```python
from build123d import *

# Parameters (mm, degrees)
SKETCH_W     = 58
SKETCH_H     = 40
PAD_DEPTH    = 2
SKETCH001_R  = 1.5
PAD001_DEPTH = 2
FILLET_R     = 3
SKETCH002_R  = 1.5
PAD002_DEPTH = 2
FILLET001_R  = 3


with BuildPart() as part:
    # Sketch → Pad (new body)
    with BuildSketch(Plane.XY):
        Rectangle(SKETCH_W, SKETCH_H)
    extrude(amount=PAD_DEPTH)

    # Sketch001 (on Face4 of Pad) → Pad001 (join)
    with BuildSketch(Plane(origin=(-29, 0, 0), x_dir=(0, -1, 0), z_dir=(-1, 0, 0))):
        with BuildLine():
            Line((-32.5, 2), (32.5, 2))
            ThreePointArc((32.5, -8), (37.5, -3), (32.5, 2))
            Line((-32.5, -8), (32.5, -8))
            ThreePointArc((-32.5, 2), (-37.5, -3), (-32.5, -8))
        make_face()
        with Locations((-32.5, -3)):
            Circle(SKETCH001_R, mode=Mode.SUBTRACT)
        with Locations((32.5, -3)):
            Circle(SKETCH001_R, mode=Mode.SUBTRACT)
    extrude(amount=PAD001_DEPTH)

    # Fillet
    fillet_edges = [part.edges().sort_by_distance(p)[0] for p in [
        (-29, 0, 0),
    ]]
    fillet(fillet_edges, radius=FILLET_R)

    # Sketch002 (on Face12 of Fillet) → Pad002 (join)
    with BuildSketch(Plane.YZ.offset(29)):
        with BuildLine():
            Line((-32.5, 2), (32.5, 2))
            ThreePointArc((32.5, -8), (37.5, -3), (32.5, 2))
            Line((-32.5, -8), (32.5, -8))
            ThreePointArc((-32.5, 2), (-37.5, -3), (-32.5, -8))
        make_face()
        with Locations((-32.5, -3)):
            Circle(SKETCH002_R, mode=Mode.SUBTRACT)
        with Locations((32.5, -3)):
            Circle(SKETCH002_R, mode=Mode.SUBTRACT)
    extrude(amount=PAD002_DEPTH)

    # Fillet001
    fillet001_edges = [part.edges().sort_by_distance(p)[0] for p in [
        (29, 0, 0),
    ]]
    fillet(fillet001_edges, radius=FILLET001_R)


solid = part.part
```
Geometry: final body of the model. Coordinates: model frame, mm. A direction names the side the tool comes from. Round coordinates to 2 decimals unless told otherwise and drop trailing zeros. Loops run counter-clockwise (first coordinate to the right, second up) from the corner with the lowest first, then second, coordinate; pieces in that order, holes last. Notation, with made-up numbers: (54.5, 27.5) -> (105.5, 27.5) arc R14 ccw to (105.5, 41.5) -> close; hole circle Ø2 at (39.5, 64.5). An arc over 180 degrees is marked (long way). Write each question's results on one line, items separated by ' | '.
Item 1: Set-up query: faces 1 (the face through (-30, -37.5, -3.1)), 2 (the face through (29, 1, -4)), 3 (the face through (0, 20, 1)), 4 (the face through (-28.14, 0.28, -0.9)). Return all of +Z, -Z, +X, -X, +Y, -Y with unobstructed straight access to the full face (end or side cutting, diameter ignored); none if empty.
Answers below:
face 1: +X, -X, -Y | face 2: -Z | face 3: +Z, -Z, +Y | face 4: -Z, +Y, -Y
Item 2: Cut plane A-A on y = 21.5. Return the cut outline in (x, z).
Answers below:
outline: (-31, -8) -> (-29, -8) -> (-29, 2) -> (-31, 2) -> close; (29, -8) -> (31, -8) -> (31, 2) -> (29, 2) -> close
Item 3: Line query: probe 1 along X at (y, z) = (12, -6); probe 2 along Z at (x, y) = (30.35, -32.5); probe 3 along Z at (x, y) = (2, -1). Output: solid intervals per line, ascending. Write a range as [from, to].
Answers below:
probe 1: x = [-31, -29], [29, 31] | probe 2: z = [-8, -4.5], [-1.5, 2] | probe 3: z = [0, 2]
Item 4: Pull-direction query (Z, two-part tool) for faces 5 (the face through (30, -37.5, -2.9)), 6 (the face through (0, -20, 1)), 7 (the face through (30, -34, -3)); classes: pulls with the +Z half, pulls with the -Z half, needs draft (parallel to the pull), parting line crosses it, or undercut.
Answers below:
face 5: parting line crosses it | face 6: needs draft | face 7: undercut
Item 5: Cut plane C-C on y = -11. Return the cut outline in (x, z), and give its area (3 significant figures).
Answers below:
outline: (-31, -8) -> (-29, -8) -> (-29, -3) arc R3 cw to (-26, 0) -> (26, 0) arc R3 cw to (29, -3) -> (29, -8) -> (31, -8) -> (31, 2) -> (-31, 2) -> close | area: 160 mm²
Item 6: Cut plane B-B on z = -5.5. Return the cut outline in (x, y), and give its area (3 significant figures).
Answers below:
outline: (-31, -36.83) -> (-29, -36.83) -> (-29, 36.83) -> (-31, 36.83) -> close; (29, -36.83) -> (31, -36.83) -> (31, 36.83) -> (29, 36.83) -> close | area: 295 mm²
Item 7: Cut plane D-D on x = 4.5. Return the cut outline in (y, z), and give its area (3 significant figures).
Answers below:
outline: (-20, 0) -> (20, 0) -> (20, 2) -> (-20, 2) -> close | area: 80.0 mm²
Item 8: Pin query (flat end, axial travel): pin 1 Ø2 at (x, y) = (17.5, 16.5) entering from -Z; pin 2 Ø2.5 at (x, z) = (-4, -0.5) entering from +Y; pin 3 Ø5.5 at (x, z) = (7.5, -1) entering from -Y. Return the tip coordinate at first contact, or that it passes through.
Answers below:
pin 1: stops at z = 0 | pin 2: stops at y = 20 | pin 3: stops at y = -20
